Can you work these out from the model? Positions are in its coordinate system, mm. Coordinates: 2 decimals unless noted, no trailing zeros. Order: outer loops, then holes, each group sorted by start corner. A loop starts at its lowest first (then second) coordinate and runs counter-clockwise, first axis right, second up. Notation, with made-up numbers: (53.5, 53.5) -> (83.5, 53.5) arc R23 ccw to (83.5, 61.5) -> close; hole circle Ø9 at (13, 9). An arc over 180 degrees is marked (long way). Answer in a Markdown table with one row per item.
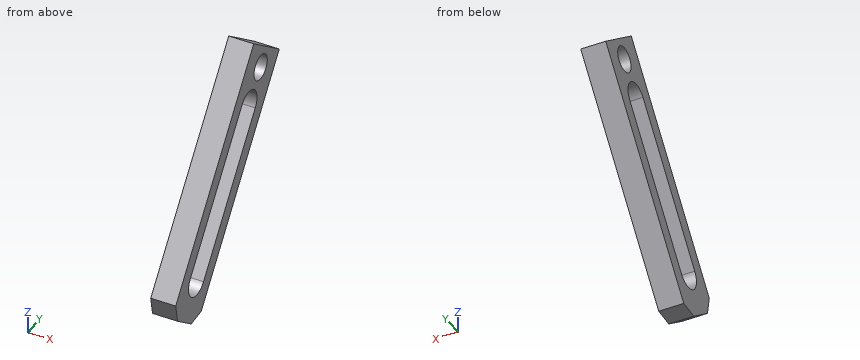
```python
from build123d import *

# Parameters (mm, degrees)
SKETCH1_R           = 8.100025456
BOSS_EXTRUDE1_DEPTH = 15.972282


with BuildPart() as part:
    # Sketch1 → Boss-Extrude1 (new body)
    with BuildSketch(Plane(origin=(0, 0, 0), x_dir=(0, 0, -1), z_dir=(1, 0, 0))):
        Polygon((253.669292, 98.434652), (277.738586, 129.464308), (400.07286, 34.572448), (400.988022, 22.300438), (394.552932, 14.004036), (388.117588, 5.707888), (376.003566, 3.542538), align=None)
        with Locations((275.620988, 106.805984)):
            Circle(SKETCH1_R, mode=Mode.SUBTRACT)
        with BuildLine():
            Line((287.497774, 84.130896), (368.581432, 21.235924))
            ThreePointArc((368.581432, 21.235924), (382.898018562, 23.044528237), (381.089408, 37.361114))
            Line((381.089408, 37.361114), (300.00575, 100.255832))
            ThreePointArc((300.00575, 100.255832), (285.689367711, 98.447294823), (287.497774, 84.130896))
        make_face(mode=Mode.SUBTRACT)
    extrude(amount=-BOSS_EXTRUDE1_DEPTH)


solid = part.part
```
(1) I need wall thicknesses on line 1 (Z direction, x = -13, y = 111.5); line 2 (Z direction, x = -14.75, y = 70); line 3 (Y direction, x = -11, z = -276.5). Which ranges of each line are inside material? Lowest first, please. Write a range as [from, to].
Response values:
| item | result |
|---|---|
| line 1 | [-300.9, -282.22], [-269.02, -263.8] |
| line 2 | [-354.4, -339.01], [-305.72, -290.33] |
| line 3 | [80.73, 98.75], [114.86, 127.87] |
(2) Suppose I cut it at A-A (y = 57). Please give me the cut outline in (x, z), and give its area (3 significant figures).
Response values:
| item | result |
|---|---|
| outline | (-15.97, -371.16) -> (0, -371.16) -> (0, -355.77) -> (-15.97, -355.77) -> close; (-15.97, -322.47) -> (0, -322.47) -> (0, -307.09) -> (-15.97, -307.09) -> close |
| area | 492 mm2 |
(3) Will these pins go through, and if not, where does the flat tip stop? pin 1 Ø8 at (x, z) = (-11.5, -367) entering from +Y; pin 2 Ø2 at (x, y) = (-6.5, 41) entering from -Z; pin 3 Ø1 at (x, y) = (-2.5, 116) entering from -Z.
Response values:
| item | result |
|---|---|
| pin 1 | y = 63.33 |
| pin 2 | z = -393.08 |
| pin 3 | z = -295.74 |
(4) Suppose I cut it at C-C (x = -4). Please give me the cut outline in (y, z), and give its area (3 significant figures).
Response values:
| item | result |
|---|---|
| outline | (3.54, -376) -> (5.71, -388.12) -> (14, -394.55) -> (22.3, -400.99) -> (34.57, -400.07) -> (129.46, -277.74) -> (98.43, -253.67) -> close; hole (21.24, -368.58) arc R10.2 ccw to (37.36, -381.09) -> (100.26, -300.01) arc R10.2 ccw to (84.13, -287.5) -> close; hole circle Ø16.2 at (106.81, -275.62) |
| area | 3,700 mm2 |
(5) Suppose I cut it at B-B (z = -350). Please give me the cut outline in (x, y), and give its area (3 significant figures).
Response values:
| item | result |
|---|---|
| outline | (-15.97, 23.71) -> (0, 23.71) -> (0, 35.65) -> (-15.97, 35.65) -> close; (-15.97, 61.48) -> (0, 61.48) -> (0, 73.41) -> (-15.97, 73.41) -> close |
| area | 381 mm2 |
